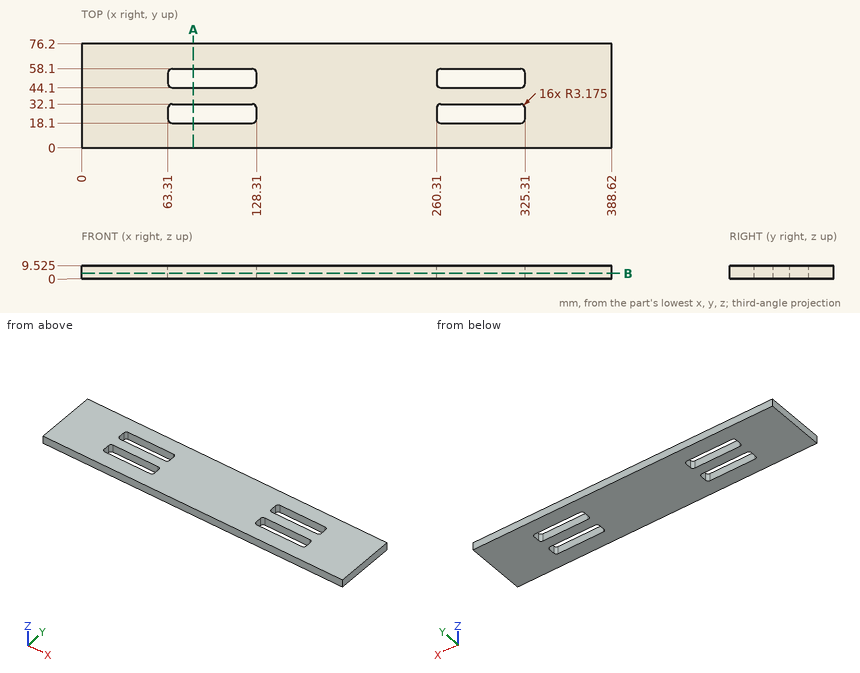
Geometry check sheet. Reference: drawing and pictorial views, mm from the part's lowest x, y, z. Round coordinates to 2 decimals unless told otherwise and drop trailing zeros. Loops run counter-clockwise (first coordinate to the right, second up) from the corner with the lowest first, then second, coordinate; pieces in that order, holes last. Notation, with made-up numbers: (57, 63) -> (79, 63) arc R22 cw to (79, 81) -> close; hole circle Ø4 at (65, 48). An arc over 180 degrees is marked (long way). Use a Markdown table: item, result.
(1) Sectioned sample at A-A (x = 82). Enter the section's corners in (y, z) (3 decimals).
Calculated:
| item | result |
|---|---|
| outline | (0, 0) -> (18.1, 0) -> (18.1, 9.525) -> (0, 9.525) -> close; (32.1, 0) -> (44.1, 0) -> (44.1, 9.525) -> (32.1, 9.525) -> close; (58.1, 0) -> (76.2, 0) -> (76.2, 9.525) -> (58.1, 9.525) -> close |
(2) Scan lines: probe 1 along X at (y, z) = (52, 2.5); probe 2 along X at (y, z) = (29.5, 6.75); probe 3 along Y at (x, z) = (81, 7.25). Record each from-to range of solid material in increasing order.
Calculated:
| item | result |
|---|---|
| probe 1 | 0 to 63.31, 128.31 to 260.31, 325.31 to 388.62 |
| probe 2 | 0 to 63.36, 128.26 to 260.36, 325.26 to 388.62 |
| probe 3 | 0 to 18.1, 32.1 to 44.1, 58.1 to 76.2 |
(3) Sectioned sample at B-B (z = 4). Give the number of separate pieces and of enclosed holes in the cut face, then the cut area to 3 significant figures.
Calculated:
| item | result |
|---|---|
| separate pieces | 1 |
| enclosed holes | 4 |
| area | 26,000 mm² |
